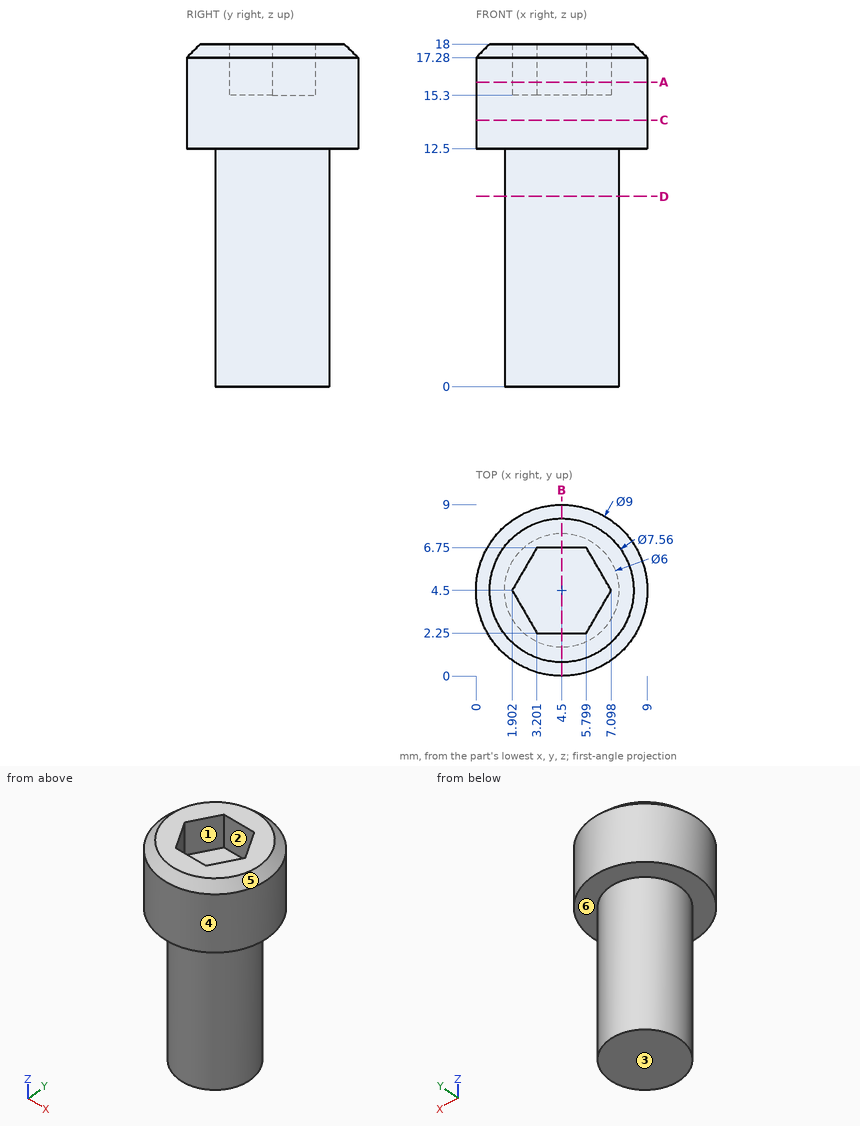
Source: three-view drawing plus pictorial views. Frame: mm from the lowest corner of the part. A direction names the side the tool comes from. Round coordinates to 2 decimals unless told otherwise and drop trailing zeros. Loops run counter-clockwise (first coordinate to the right, second up) from the corner with the lowest first, then second, coordinate; pieces in that order, holes last. Notation, with made-up numbers: (4, -4.75) - (13, -4.75) arc R25 ccw to (13, 12.25) - close; hole circle Ø6 at (-16.5, 79). An arc over 180 degrees is marked (long way). Write each question's results on one line, items separated by ' | '. Start each with the question number.
1) Mould query, pull axis Y, two halves, no side actions, for the marked faces 1, 2, 3 and 4. Classes: released by +Y, released by -Y, zero draft, split by the parting line, or undercut.
2) Cut plane D-D on z = 10. Return loops of the section in (x, y), then the cut area to 3 significant figures.
3) Line query: probe 1 along Z at (x, y) = (2.5, 7.5); probe 2 along Y at (x, z) = (6.25, 15.75); probe 3 along Y at (x, z) = (3, 5). Output: solid intervals per line, ascending. Write a range as [from, to].
4) Cut plane C-C on z = 14. Return loops of the section in (x, y).
5) Cut plane B-B on x = 4.5. Return loops of the section in (y, z), then the cut area to 3 significant figures.
6) Cut plane A-A on z = 16. Return loops of the section in (x, y).
7) Access query for the marked faces 5 and 6. Directions: +Z, -Z, +X, -X, +Y, -Y. A direction counts if a zero-diameter tool reaches every point of the face in a straight line with its end or side. Return the directions, or none.
8) First-contact query: P1, Ø2, axis at x = 6, z = 11, coming from the -Y side; P2, Ø1, axis at y = 6.5, z = 15, coming from the -X side. Flat tips, straight axial feed; report the tip coordinate or a pass-through.
Verdict:
1) face 1: undercut | face 2: undercut | face 3: zero draft | face 4: split by the parting line
2) outline: circle Ø6 at (4.5, 4.5) | area: 28.3 mm2
3) probe 1: z = [12.5, 18] | probe 2: y = [0.35, 3.03], [5.97, 8.65] | probe 3: y = [1.9, 7.1]
4) outline: circle Ø9 at (4.5, 4.5)
5) outline: (0, 12.5) - (1.5, 12.5) - (1.5, 0) - (7.5, 0) - (7.5, 12.5) - (9, 12.5) - (9, 17.28) - (8.28, 18) - (6.75, 18) - (6.75, 15.3) - (2.25, 15.3) - (2.25, 18) - (0.72, 18) - (0, 17.28) - close | area: 112 mm2
6) outline: circle Ø9 at (4.5, 4.5); hole (1.9, 4.5) - (3.2, 2.25) - (5.8, 2.25) - (7.1, 4.5) - (5.8, 6.75) - (3.2, 6.75) - close
7) face 5: +Z | face 6: -Z
8) P1: stops at y = 1.54 | P2: stops at x = 0.26
